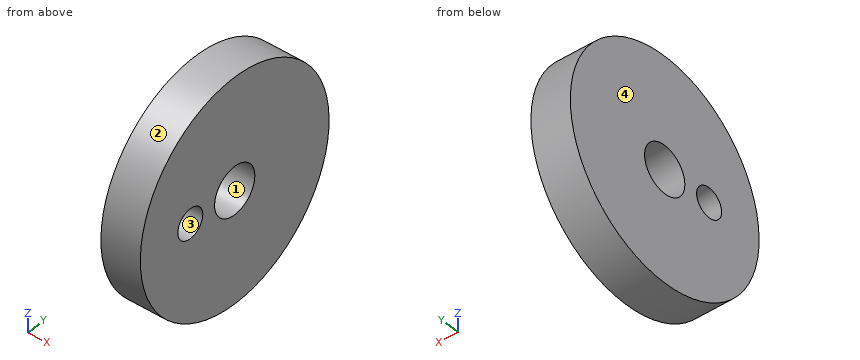
from build123d import *

# Parameters (mm, degrees)
SKETCH1_R                 = 34
BOSS_EXTRUDE1_DEPTH       = 12
M13_CLEARANCE_HOLE1_D     = 14.5
M13_CLEARANCE_HOLE1_DEPTH = 30
M13_CLEARANCE_HOLE1_TIP   = 4.356239488
M8_CLEARANCE_HOLE1_D      = 9
M8_CLEARANCE_HOLE1_DEPTH  = 30
M8_CLEARANCE_HOLE1_TIP    = 2.703872786


with BuildPart() as part:
    # Sketch1 → Boss-Extrude1 (new body)
    with BuildSketch(Plane(origin=(0, 0, 0), x_dir=(0, 0, -1), z_dir=(1, 0, 0))):
        Circle(SKETCH1_R)
    extrude(amount=BOSS_EXTRUDE1_DEPTH)

    # M13 Clearance Hole1
    with Locations(Plane(origin=(12, 0, 0), x_dir=(0, 0, -1), z_dir=(1, 0, 0))):
        with Locations((0, 0)):
            Hole(M13_CLEARANCE_HOLE1_D / 2, depth=M13_CLEARANCE_HOLE1_DEPTH)
            with Locations((0, 0, -(M13_CLEARANCE_HOLE1_DEPTH + M13_CLEARANCE_HOLE1_TIP / 2))):  # 118° drill point
                Cone(0, M13_CLEARANCE_HOLE1_D / 2, M13_CLEARANCE_HOLE1_TIP, mode=Mode.SUBTRACT)

    # M8 Clearance Hole1
    with Locations(Plane(origin=(12, 0, 0), x_dir=(0, 0, -1), z_dir=(1, 0, 0))):
        with Locations((0, -16)):
            Hole(M8_CLEARANCE_HOLE1_D / 2, depth=M8_CLEARANCE_HOLE1_DEPTH)
            with Locations((0, 0, -(M8_CLEARANCE_HOLE1_DEPTH + M8_CLEARANCE_HOLE1_TIP / 2))):  # 118° drill point
                Cone(0, M8_CLEARANCE_HOLE1_D / 2, M8_CLEARANCE_HOLE1_TIP, mode=Mode.SUBTRACT)


solid = part.part
Can you work these out from the model? Positions are in its coordinate system, mm. Face numbers are marked on the shaded views. Coordinates: 2 decimals unless noted, no trailing zeros. Write each loop counter-clockwise with the first axis right and the second up, starting at its lowest first coordinate (ties: lowest second). Pieces come first, ordered by that corner, then holes. Notation, with made-up numbers: (-11.5, 2.5) - (1.5, 2.5) arc R24 ccw to (1.5, 21.5) - close; hole circle Ø3 at (3.5, 14). An arc over 180 degrees is marked (long way). Return JSON: item names as keys, results as strings. Group by question number.
Item 1: We'd pull the mould along Z, two halves only. Please class the marked faces 1, 2, 3 and 4: pulls with the +Z half, pulls with the -Z half, needs draft (parallel to the pull), parting line crosses it, or undercut.
Item 2: I'm going to push flat-ended pins straight in: pin 1 Ø3 at (x, z) = (3, 23.5) entering from +Y; pin 2 Ø5 at (y, z) = (1, -3) entering from +X; pin 3 Ø5 at (x, y) = (4.5, -24) entering from +Z. Where does each tip first touch, or does it pass through?
Item 3: If we section it at D-D (y = 0): Write out the boundary of the cut face in (x, z), then the cut area to 3 significant figures.
Item 4: If we section it at C-C (x = 2): Write out the boundary of the cut face in (y, z), then the cut area to 3 significant figures.
Item 5: If we section it at B-B (y = -16): Write out the boundary of the cut face in (x, z), then the cut area to 3 significant figures.
Item 6: Please list where these lines run through material, in increasing order: probe 1 along Y at (x, z) = (7.25, 0); probe 2 along Y at (x, z) = (6.75, 1.5); probe 3 along Z at (x, y) = (2.5, -20).
Item 7: If we section it at A-A (z = 0): Write out the boundary of the cut face in (x, y).
Return value:
{
 "1": {"face 1": "undercut", "face 2": "parting line crosses it", "face 3": "undercut", "face 4": "needs draft"},
 "2": {"pin 1": "stops at y = 25.92", "pin 2": "passes through", "pin 3": "stops at z = 26.34"},
 "3": {"outline": "(0, -34) - (12, -34) - (12, -7.25) - (0, -7.25) - close; (0, 7.25) - (12, 7.25) - (12, 34) - (0, 34) - close", "area": "642 mm^2"},
 "4": {"outline": "circle Ø68 at (0, 0); hole circle Ø9 at (-16, 0); hole circle Ø14.5 at (0, 0)", "area": "3,400 mm^2"},
 "5": {"outline": "(0, -30) - (12, -30) - (12, -4.5) - (0, -4.5) - close; (0, 4.5) - (12, 4.5) - (12, 30) - (0, 30) - close", "area": "612 mm^2"},
 "6": {"probe 1": "y = -34 to -20.5, -11.5 to -7.25, 7.25 to 34", "probe 2": "y = -33.97 to -20.24, -11.76 to -7.09, 7.09 to 33.97", "probe 3": "z = -27.5 to -2.06, 2.06 to 27.5"},
 "7": {"outline": "(0, -34) - (12, -34) - (12, -20.5) - (0, -20.5) - close; (0, -11.5) - (12, -11.5) - (12, -7.25) - (0, -7.25) - close; (0, 7.25) - (12, 7.25) - (12, 34) - (0, 34) - close"}
}
